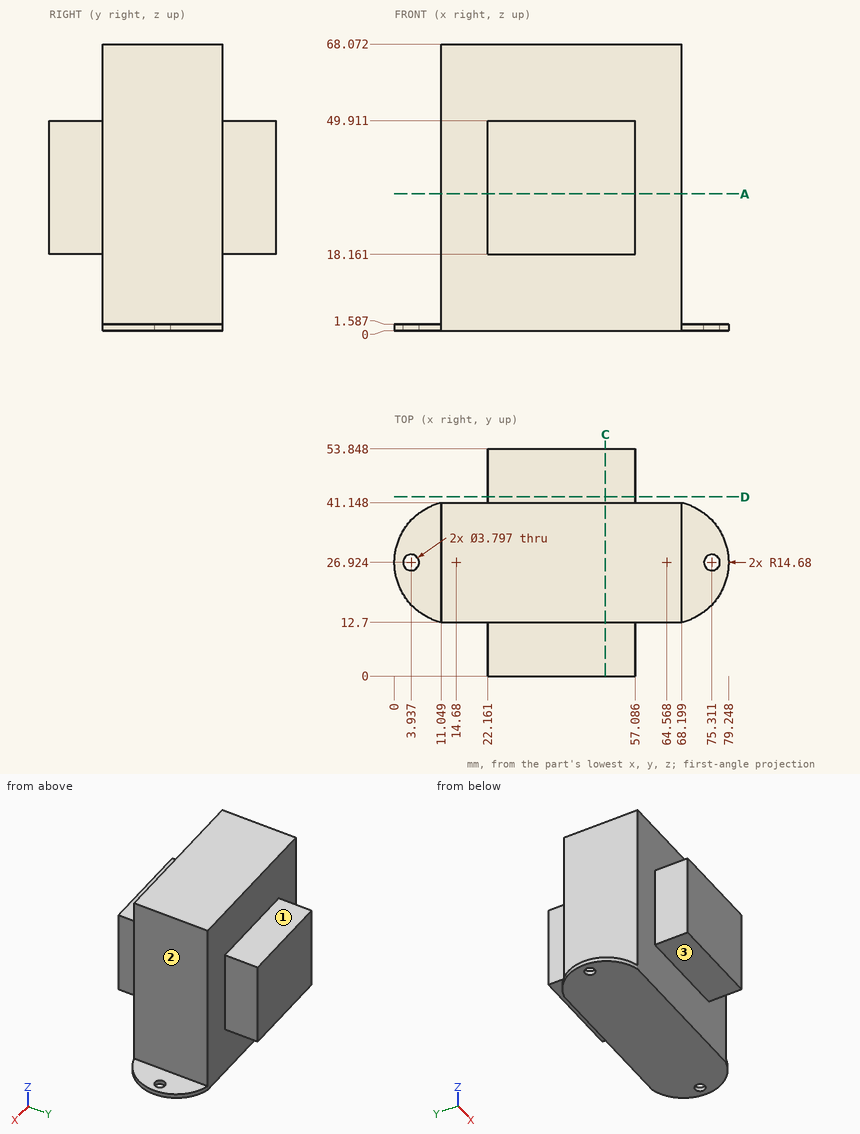
The figure shows three views and two pictorial views of one solid part (mm, origin at its lowest corner). Answer the questions. A direction names the side the tool comes from. Give positions to 0.01 mm unless a question says otherwise; leave off trailing zeros. Write each loop counter-clockwise with the first axis right and the second up, starting at its lowest first coordinate (ties: lowest second). Pieces come first, ordered by that corner, then holes. Notation, with made-up numbers: (-29.75, 0.25) - (18.25, 0.25) arc R30 ccw to (18.25, 38.25) - close; hole circle Ø4 at (-27, 4.25). An arc over 180 degrees is marked (long way). Use CSV: the item, a comma, the result in double quotes. Start each with the question number.
Item 1: The part is cut by section A-A, the plane z = 32.5. Give the vertices of the cut face in (x, y), and give its area (3 significant figures).
Item 2: Flat-ended cylindrical pins translate along their axes: P1, Ø10, axis at y = 5, z = 31, coming from the +X side; P2, Ø10, axis at x = 40.5, z = 14.5, coming from the -Y side; P3, Ø10, axis at y = 45.5, z = 36, coming from the -X side; P4, Ø3, axis at x = 75.311, y = 26.924, coming from the -Z side. Find the tip coordinate at first contact, or state that the pin passes through.
Item 3: For the marked faces 1, 2 and 3, determine the directions among +Z, -Z, +X, -X, +Y, -Y from which every point of the face is accessible in a straight line to the end or side of a thin tool.
Item 4: Consider line 1 (Z direction, x = 8, y = 35); line 2 (X direction, y = 36.5, z = 43); line 3 (Y direction, x = 67, z = 46.5). Determine where each line is inside the solid, lowest interval first.
Item 5: The part is cut by section D-D, the plane y = 42.5. Give the vertices of the cut face in (x, z).
Item 6: The part is cut by section C-C, the plane x = 50. Give the vertices of the cut face in (y, z), and give its area (3 significant figures).
Taken from the geometry:
1,outline,"(11.05, 12.7) - (22.16, 12.7) - (22.16, 0) - (57.09, 0) - (57.09, 12.7) - (68.2, 12.7) - (68.2, 41.15) - (57.09, 41.15) - (57.09, 53.85) - (22.16, 53.85) - (22.16, 41.15) - (11.05, 41.15) - close"
1,area,"2,510 mm2"
2,P1,"x = 57.09"
2,P2,"y = 0"
2,P3,"x = 11.05"
2,P4,"through"
3,face 1,"+Z, +X, -X, +Y"
3,face 2,"+Z, +X, +Y, -Y"
3,face 3,"-Z, +X, -X, -Y"
4,line 1,"0 to 1.59"
4,line 2,"11.05 to 68.2"
4,line 3,"12.7 to 41.15"
5,outline,"(22.16, 18.16) - (57.09, 18.16) - (57.09, 49.91) - (22.16, 49.91) - close"
6,outline,"(0, 18.16) - (12.7, 18.16) - (12.7, 0) - (41.15, 0) - (41.15, 18.16) - (53.85, 18.16) - (53.85, 49.91) - (41.15, 49.91) - (41.15, 68.07) - (12.7, 68.07) - (12.7, 49.91) - (0, 49.91) - close"
6,area,"2,740 mm2"
